Print and shaded views of the part. All mm, measured from the part's lowest x, y and z. A direction names the side the tool comes from. Round coordinates to 2 decimals unless told otherwise and drop trailing zeros. Loops run counter-clockwise (first coordinate to the right, second up) from the corner with the lowest first, then second, coordinate; pieces in that order, holes last. Notation, with made-up numbers: (-13.5, 78.25) -> (34.5, 78.25) arc R26 ccw to (34.5, 107.25) -> close; hole circle Ø6 at (-36, 69). An arc over 180 degrees is marked (long way). Use a Markdown table: item, result.
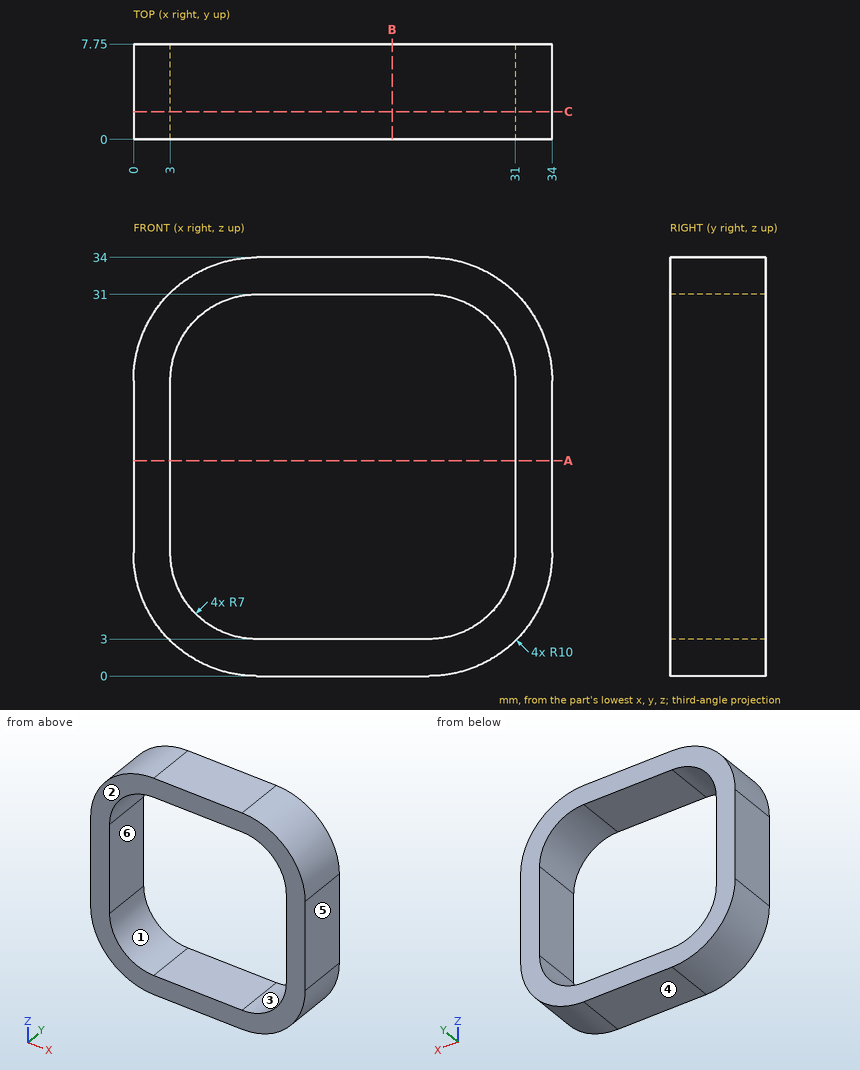
Q1. Drill centre lines: L1, parallel to Z at x = 15, y = 5.75; L2, parallel to X at y = 1.5, z = 28. Where is each one in solid material? Low to high. Write a range as from..to.
Results list:
| item | result |
|---|---|
| L1 | z = 0..3, 31..34 |
| L2 | x = 0.83..4.26, 29.74..33.17 |
Q2. Tool access for the marked faces 1 and 2: list every direction of +Z, -Z, +X, -X, +Y, -Y with a clear straight run to the whole face (end or side of a thin tool).
Results list:
| item | result |
|---|---|
| face 1 | +Y, -Y |
| face 2 | +Z, -Z, +X, -X, -Y |
Q3. Flat gauge pin, fed straight in: pin 1 (4 mm diameter, centred on x = 27.5, y = 5.5, fed in from -Z). Where does the tip first touch, or does it go through?
Results list:
| item | result |
|---|---|
| pin 1 | stops at z = 0.11 |
Q4. Pull direction X, two halves, no side cores. Call the marked faces 3, 4, 5 and 6: released by +X, released by -X, zero draft, split by the parting line, or undercut.
Results list:
| item | result |
|---|---|
| face 3 | undercut |
| face 4 | zero draft |
| face 5 | released by +X |
| face 6 | undercut |
Q5. Band-saw the part on B-B, the plane x = 21. Give the cut face in (y, z).
Results list:
| item | result |
|---|---|
| outline | (0, 0) -> (7.75, 0) -> (7.75, 3) -> (0, 3) -> close; (0, 31) -> (7.75, 31) -> (7.75, 34) -> (0, 34) -> close |
Q6. Band-saw the part on A-A, the plane z = 17.5. Give the cut face in (x, y).
Results list:
| item | result |
|---|---|
| outline | (0, 0) -> (3, 0) -> (3, 7.75) -> (0, 7.75) -> close; (31, 0) -> (34, 0) -> (34, 7.75) -> (31, 7.75) -> close |
Q7. Band-saw the part on C-C, the plane y = 2.25. Give the cut face in (x, z), plus the area to 3 significant figures.
Results list:
| item | result |
|---|---|
| outline | (0, 10) arc R10 ccw to (10, 0) -> (24, 0) arc R10 ccw to (34, 10) -> (34, 24) arc R10 ccw to (24, 34) -> (10, 34) arc R10 ccw to (0, 24) -> close; hole (3, 10) arc R7 ccw to (10, 3) -> (24, 3) arc R7 ccw to (31, 10) -> (31, 24) arc R7 ccw to (24, 31) -> (10, 31) arc R7 ccw to (3, 24) -> close |
| area | 328 mm² |
